Check sheet for the modelled part. Datum: model origin and axes. Units: mm. Coordinates: 2 decimals unless noted, no trailing zeros. Loops run counter-clockwise (first coordinate to the right, second up) from the corner with the lowest first, then second, coordinate; pieces in that order, holes last. Notation, with made-up numbers: (56.5, 26) -> (84.5, 26) arc R32 cw to (84.5, 65) -> close; hole circle Ø4 at (-33.75, -1). An arc over 180 degrees is marked (long way). Use one line per item in the form item = value.
from build123d import *

# Parameters (mm, degrees)
EXTRUDE_1_DEPTH     = 3
SKETCH_2_W          = 55
SKETCH_2_H          = 3
CUT_EXTRUDE_1_DEPTH = 86.300937861
EXTRUDE_2_DEPTH     = 3
FILLET_1_R          = 10
SKETCH_4_R          = 1.6
SKETCH_4_W          = 30
SKETCH_4_H          = 6
CUT_EXTRUDE_2_DEPTH = 86.581832184
FILLET_2_R          = 1


with BuildPart() as part:
    # 草图1 → 凸台-拉伸1 (new body)
    with BuildSketch(Plane.XY):
        Polygon((-85, 1), (-85, 3.5), (-70.5, 3.5), (-70.5, 6.5), (-60.5, 6.5), (-60.5, 3.5), (-27.5, 3.5), (-27.5, 6.5), (-17.5, 6.5), (-17.5, 3.5), (17.5, 3.5), (17.5, 6.5), (27.5, 6.5), (27.5, 3.5), (60.5, 3.5), (60.5, 6.5), (70.5, 6.5), (70.5, 3.5), (85, 3.5), (85, 1), (79, 1), (79, 0), (-79, 0), (-79, 1), align=None)
    extrude(amount=EXTRUDE_1_DEPTH)

    # 草图2 → 切除-拉伸1 (cut, through all)
    with BuildSketch(Plane.XY.offset(3)):
        with Locations((0, 5)):
            Rectangle(SKETCH_2_W, SKETCH_2_H)
    extrude(amount=-CUT_EXTRUDE_1_DEPTH, mode=Mode.SUBTRACT)

    # 草图3 → 凸台-拉伸2 (add)
    with BuildSketch(Plane.XY.offset(3)):
        Polygon((-50, 0), (50, 0), (59.5, 0), (50, -9.5), (-50, -9.5), (-59.5, 0), align=None)
    extrude(amount=-EXTRUDE_2_DEPTH)

    # 圆角1
    fillet_1_edges = [part.edges().sort_by_distance(p)[0] for p in [
        (-59.5, 0, 1.5),
        (59.5, 0, 1.5),
        (50, -9.5, 1.5),
        (-50, -9.5, 1.5),
    ]]
    fillet(fillet_1_edges, radius=FILLET_1_R)

    # 草图4 → 切除-拉伸2 (cut, through all)
    with BuildSketch(Plane.XY.offset(3)):
        with Locations((-22.5, -2.5)):
            Circle(SKETCH_4_R)
        with Locations((22.5, -2.5)):
            Circle(SKETCH_4_R)
        Polygon((-49.1, 3.5), (-45.9, 3.5), (-45.9, -1), (-44.5, -1), (-44.5, -4), (-45.9, -4), (-45.9, -5.5), (-49.1, -5.5), (-49.1, -4), (-50.5, -4), (-50.5, -1), (-49.1, -1), align=None)
        Polygon((50.5, -1), (49.1, -1), (49.1, 3.5), (45.9, 3.5), (45.9, -1), (44.5, -1), (44.5, -4), (45.9, -4), (45.9, -5.5), (49.1, -5.5), (49.1, -4), (50.5, -4), align=None)
        with Locations((0, -6.5)):
            Rectangle(SKETCH_4_W, SKETCH_4_H)
    extrude(amount=-CUT_EXTRUDE_2_DEPTH, mode=Mode.SUBTRACT)

    # 圆角2
    fillet_2_edges = [part.edges().sort_by_distance(p)[0] for p in [
        (-15, -9.5, 1.5),
        (-15, -3.5, 1.5),
        (15, -3.5, 1.5),
        (15, -9.5, 1.5),
    ]]
    fillet(fillet_2_edges, radius=FILLET_2_R)


solid = part.part
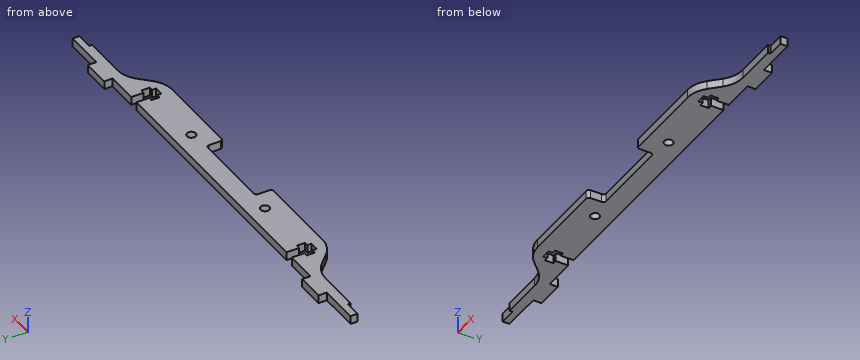
(1) Section check A-A, the plane x = -22.5. Record the boundary of the cut face in (y, z).
Established:
outline = (-9.5, 0) -> (-4.1, 0) -> (-4.1, 3) -> (-9.5, 3) -> close; (-0.9, 0) -> (3.5, 0) -> (3.5, 3) -> (-0.9, 3) -> close
(2) Scan lines: line 1 along Y through (x, z) = (22.5, 1.65); line 2 along X through (y, z) = (2, 1.5); line 3 along X through (y, z) = (5, 1.9). Record each from-to range of solid material in increasing order.
Established:
line_1 = -9.5 to -4.1, -0.9 to 3.5
line_2 = -85 to -49.1, -45.9 to 45.9, 49.1 to 85
line_3 = -70.5 to -60.5, 60.5 to 70.5
(3) Section check B-B, the plane z = 2.15. Give the number of separate pieces and of enclosed holes in the cut face, plus the area to 3 significant figures.
Established:
separate_pieces = 1
enclosed_holes = 2
area = 1,410 mm²
(4) Go/stop test with flat-tipped pins: P1, Ø1.5, axis at x = -80.5, z = 1.5, coming from the +Y side; P2, Ø0.8, axis at y = -5, z = 1.5, coming from the +X side; P3, Ø1.6, axis at y = -4.5, z = 2, coming from the +X side; P4, Ø3, axis at x = -22.5, y = -2.5, coming from the +Z side. Record where each tip stops, or that it passes through.
Established:
P1 = 3.5
P2 = 54.9
P3 = 55.8
P4 = through
(5) Section check C-C, the plane x = -68. Record the boundary of the cut face in (y, z).
Established:
outline = (0, 0) -> (6.5, 0) -> (6.5, 3) -> (0, 3) -> close
(6) Section check D-D, the plane x = -5.5. Record the boundary of the cut face in (y, z), plus the area to 3 significant figures.
Established:
outline = (-3.5, 0) -> (3.5, 0) -> (3.5, 3) -> (-3.5, 3) -> close
area = 21.0 mm²
